Autodesk Inventor part; units mm, degrees
ref_plane "YZ Plane" through (0, 0, 0) normal (1, 0, 0) x (0, 1, 0)
ref_plane "XZ Plane" through (0, 0, 0) normal (0, 1, 0) x (-1, 0, 0)
ref_plane "XY Plane" through (0, 0, 0) normal (0, 0, 1) x (1, 0, 0)
sketch "스케치1" plane through (0, 0, 0) normal (0, 1, 0) x (-1, 0, 0)
  line L0 (-13, 13) -> (13, 13)
  line L1 (13, 13) -> (13, -13)
  line L2 (13, -13) -> (-13, -13)
  line L3 (-13, -13) -> (-13, 13)
  line L4 (-13, 13) -> (13, -13) construction
  line L5 (13, 13) -> (-13, -13) construction
  circle A0 centre (11, 11) radius 1
  line L6 (12.35, -8.2) -> (-12.35, -8.2)
  line L7 (-12.35, -8.2) -> (-12.35, 8.8)
  line L8 (-12.35, 8.8) -> (12.35, 8.8)
  line L9 (12.35, 8.8) -> (12.35, -8.2)
  line L10 (12.35, 5.3) -> (-12.35, 5.3)
  line L11 (0, 0) -> (0, -5.5368) construction
  line L12 (0, 0) -> (-4.847, 0) construction
  circle A1 centre (-11, 11) radius 1
  circle A2 centre (11, -11) radius 1
  circle A3 centre (-11, -11) radius 1
  dimension "d0" = 26
  dimension "d1" = 26
  dimension "d5" = 2
  dimension "d6" = 2
  dimension "d14" = 2
  dimension "d15" = 24.7
  dimension "d16" = 17
  dimension "d17" = 4.8
  dimension "d18" = 13.5
extrude "돌출1" add sketch "스케치1" against normal blind 1 contours L0 L1 L2 L3 | L6 L7 L10 L9 | L10 L7 L8 L9
extrude "돌출3" add sketch "스케치1" along normal blind 2 contours L6 L7 L10 L9
extrude "돌출4" add sketch "스케치1" along normal blind 1.8 contours L10 L7 L8 L9
sketch "스케치2" plane through (0, 0, 0) normal (0, 1, 0) x (1, 0, 0)
  line L0 (-7, -11.5) -> (7, -11.5)
  line L1 (7, -11.5) -> (7, -14.5)
  line L2 (7, -14.5) -> (-7, -14.5)
  line L3 (-7, -14.5) -> (-7, -11.5)
  line L4 (13, -13) -> (-13, -13)
  line L5 (-7, -11.5) -> (7, -14.5) construction
  line L6 (7, -11.5) -> (-7, -14.5) construction
  point P0 (0, 0)
  point P1 (0, -13)
  dimension "d23" = 14
  dimension "d24" = 3
extrude "돌출5" cut sketch "스케치2" against normal blind 16.75
sketch "스케치3" plane through (0, 0, 0) normal (0, 1, 0) x (1, 0, 0)
  circle A0 centre (-11, 11) radius 1
  circle A1 centre (-11, 11) radius 2
  circle A2 centre (11, 11) radius 1
  circle A3 centre (11, 11) radius 2
  circle A4 centre (11, -11) radius 1
  circle A5 centre (11, -11) radius 2
  circle A6 centre (-11, -11) radius 1
  circle A7 centre (-11, -11) radius 2
  point P0 (0, 0)
  dimension "d27" = 4
extrude "돌출6" add sketch "스케치3" along normal blind 0.1
properties part number "OLED Display"
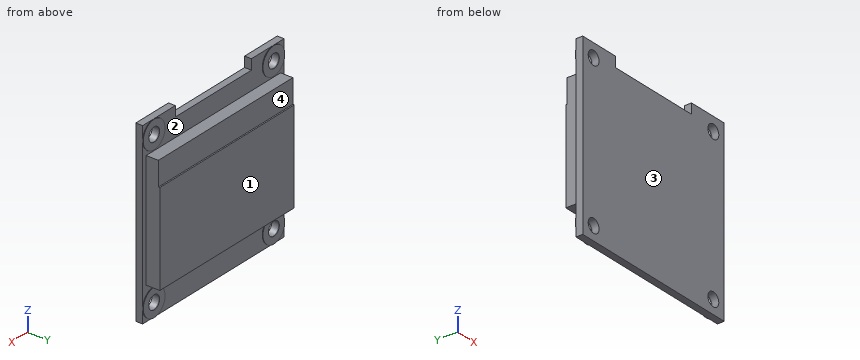
CAD build for the part. Positions are in the model's coordinates, mm. Face numbers are marked on the shaded views. A direction names the side the tool comes from. Coordinates: 2 decimals unless noted, no trailing zeros. Write each loop counter-clockwise with the first axis right and the second up, starting at its lowest first coordinate (ties: lowest second). Pieces come first, ordered by that corner, then holes. Notation, with made-up numbers: (56.25, 63.25) -> (87.25, 63.25) arc R11 ccw to (87.25, 81.25) -> close; hole circle Ø7 at (34.5, -39.75). An arc over 180 degrees is marked (long way). Return JSON: item names as keys, results as strings. Group by question number.
Q1. Cut at B-B, the plane x = 2.5. Give the cut face in (y, z).
Q2. Cut at A-A, the plane y = -0.5. Give the cut face in (x, z).
Q3. Flat gauge pins, fed straight in: pin 1 (3 mm diameter, centred on x = -10, z = -10, fed in from +Y); pin 2 (1 mm diameter, centred on x = 6, y = 1, fed in from -Z); pin 3 (1.8 mm diameter, centred on x = 1.5, z = 6.5, fed in from +Y). Where does each tip first touch, or does it go through?
Q4. Cut at D-D, the plane y = 1.05. Give the cut face in (x, z), then the cut area to 3 significant figures.
Q5. Cut at C-C, the plane z = -7.75. Give the cut face in (x, y).
Q6. Drill centre lines: line 1 (X direction, y = -0.6, z = 11); line 2 (X direction, y = 0.05, z = -11). Where is each one in solid material? Low to high.
Q7. Which spindle directions (+Z, -Z, +X, -X, +Y, -Y) get a long thin tool onto all of the face, cutting with end or side? Do the marked faces 3 and 4. Say none if no direction does.
Q8. Pull direction X, two halves, no side cores. Call the marked faces 1 and 2: released by +X, released by -X, zero draft, split by the parting line, or undercut.
Returned:
{
 "1": {"outline": "(-1, -13) -> (0, -13) -> (0, -8.2) -> (2, -8.2) -> (2, 5.3) -> (1.8, 5.3) -> (1.8, 8.8) -> (0, 8.8) -> (0, 11.5) -> (-1, 11.5) -> close"},
 "2": {"outline": "(-13, -13) -> (13, -13) -> (13, 13) -> (7, 13) -> (7, 11.5) -> (-7, 11.5) -> (-7, 13) -> (-13, 13) -> close; hole circle Ø2 at (-11, -11); hole circle Ø2 at (-11, 11); hole circle Ø2 at (11, -11); hole circle Ø2 at (11, 11)"},
 "3": {"pin 1": "stops at y = 0.1", "pin 2": "stops at z = -8.2", "pin 3": "stops at y = 1.8"},
 "4": {"outline": "(-12.35, -8.2) -> (12.35, -8.2) -> (12.35, 8.8) -> (-12.35, 8.8) -> close", "area": "420 mm2"},
 "5": {"outline": "(-13, -1) -> (13, -1) -> (13, 0) -> (12.35, 0) -> (12.35, 2) -> (-12.35, 2) -> (-12.35, 0) -> (-13, 0) -> close"},
 "6": {"line 1": "x = -13 to -12, -10 to 10, 12 to 13", "line 2": "x = -13 to -12, -10 to -9, 9 to 10, 12 to 13"},
 "7": {"face 3": "+Z, -Z, +X, -X, -Y", "face 4": "+Z, +X, -X, +Y"},
 "8": {"face 1": "zero draft", "face 2": "undercut"}
}
